Geometry: see drawing. Coordinates: mm, zero at the bounding-box minimum. A direction names the side the tool comes from. Give positions to 0.01 mm unless a question says otherwise; leave off trailing zeros. Order: outer loops, then holes, each group sorted by start corner. A loop starts at its lowest first (then second) coordinate and runs counter-clockwise, first axis right, second up. Notation, with made-up numbers: (42, 52.5) - (71, 52.5) arc R17 cw to (71, 76.5) - close; hole circle Ø8 at (75.5, 72). An arc over 180 degrees is marked (long way). Write item = value, one per line. Start each with the question number.
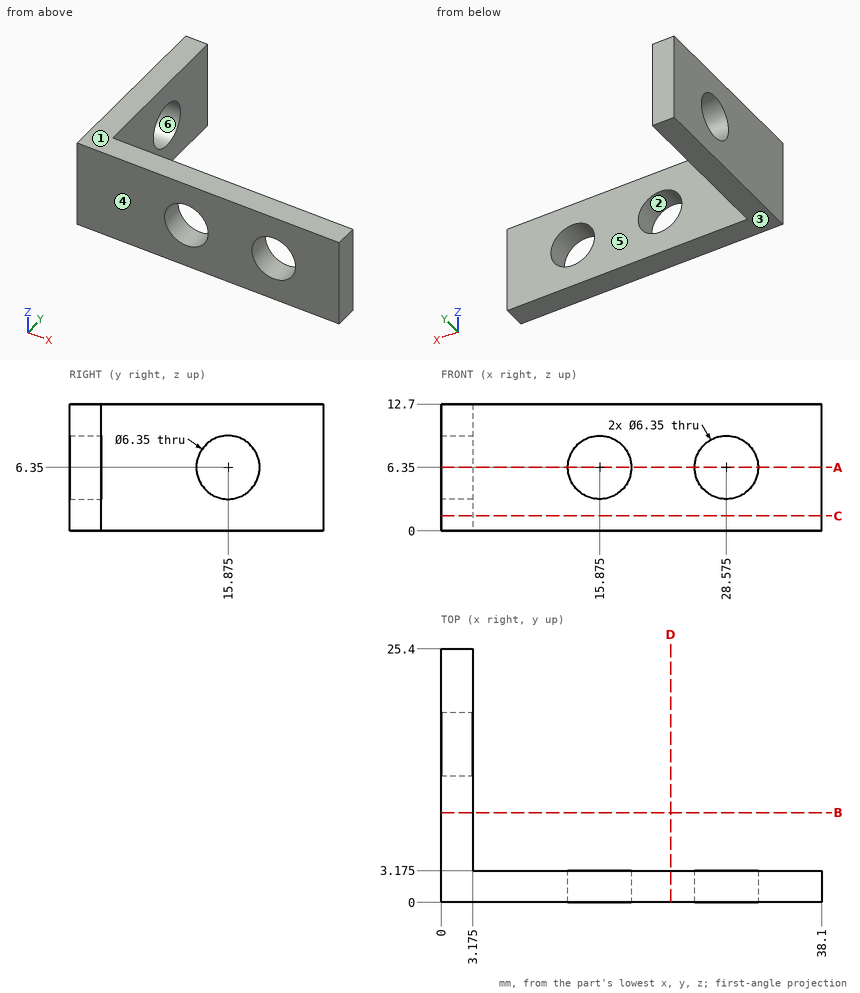
Q1. Material intervals for line 1 along X through (y, z) = (1.95, 6.35); line 2 along Y through (x, z) = (1.35, 6.35); line 3 along Z through (x, y) = (28.5, 2.75), sorted ascending. Write a range as from..to.
Q2. Section B-B, the plane y = 9. Return the cut outline in (x, z) (3 decimals), then the cut area to 3 significant figures.
Q3. Pull-direction query (Z, two-part tool) for the marked faces 1, 2, 3 and 4; classes: +Z half, -Z half, draft (parallel to the pull), parting line (faces both ways), or undercut.
Q4. Contact query for flat-ended pins moving along their axis: pin 1 (5 mm diameter, centred on y = 9, z = 11, fed in from +X) (3 decimals); pin 2 (5 mm diameter, centred on x = 18, z = 8, fed in from +Y) (3 decimals). Output: stop coordinate, or through.
Q5. Section C-C, the plane z = 1.5. Return the cut outline in (x, y) (3 decimals), then the cut area to 3 significant figures.
Q6. Section A-A, the plane z = 6.35. Return the cut outline in (x, y) (3 decimals).
Q7. Set-up query: the marked faces 5 and 6. Return all of +Z, -Z, +X, -X, +Y, -Y with unobstructed straight access to the full face (end or side cutting, diameter ignored); none if empty.
The answers:
q1.line_1 = 0..12.7, 19.05..25.4, 31.75..38.1
q1.line_2 = 0..12.7, 19.05..25.4
q1.line_3 = 0..3.18, 9.52..12.7
q2.outline = (0, 0) - (3.175, 0) - (3.175, 12.7) - (0, 12.7) - close
q2.area = 40.3 mm²
q3.face_1 = +Z half
q3.face_2 = undercut
q3.face_3 = -Z half
q3.face_4 = draft
q4.pin_1 = 3.175
q4.pin_2 = 3.175
q5.outline = (0, 0) - (38.1, 0) - (38.1, 3.175) - (3.175, 3.175) - (3.175, 25.4) - (0, 25.4) - close
q5.area = 192 mm²
q6.outline = (0, 0) - (12.7, 0) - (12.7, 3.175) - (3.175, 3.175) - (3.175, 12.7) - (0, 12.7) - close; (0, 19.05) - (3.175, 19.05) - (3.175, 25.4) - (0, 25.4) - close; (19.05, 0) - (25.4, 0) - (25.4, 3.175) - (19.05, 3.175) - close; (31.75, 0) - (38.1, 0) - (38.1, 3.175) - (31.75, 3.175) - close
q7.face_5 = +Z, -Z, +X, +Y
q7.face_6 = +X, -X
